The listing builds one solid part. Answer for the finished solid, in the listing's coordinates (mm). Face numbers are marked on the shaded views. A direction names the side the tool comes from. Coordinates: 2 decimals unless noted, no trailing zeros. Write each loop counter-clockwise with the first axis right and the second up, starting at its lowest first coordinate (ties: lowest second). Pieces come first, ordered by that corner, then holes.
from build123d import *

# Parameters (mm, degrees)
SKETCH1_W           = 200
SKETCH1_H           = 200
BOSS_EXTRUDE1_DEPTH = 5.6
SKETCH2_W           = 200
SKETCH2_H           = 200
SKETCH2_W_2         = 188.8
SKETCH2_H_2         = 188.8
BOSS_EXTRUDE2_DEPTH = 136
SKETCH3_W           = 5.6
SKETCH3_H           = 30.4
BOSS_EXTRUDE3_DEPTH = 32
FILLET1_R           = 25
SKETCH4_R           = 110
CUT_EXTRUDE1_DEPTH  = 12
FILLET3_R           = 10
FILLET2_R           = 2.4
SKETCH5_W           = 12
SKETCH5_H           = 12
BOSS_EXTRUDE4_DEPTH = 88
FILLET4_R           = 5
SKETCH6_R           = 1.55
CUT_EXTRUDE2_DEPTH  = 332.868889774
FILLET5_R           = 1.6


with BuildPart() as part:
    # Sketch1 → Boss-Extrude1 (new body)
    with BuildSketch(Plane(origin=(0, 0, 0), x_dir=(1, 0, 0), z_dir=(0, 1, 0))):
        with Locations((100, -100)):
            Rectangle(SKETCH1_W, SKETCH1_H)
    extrude(amount=BOSS_EXTRUDE1_DEPTH)

    # Sketch2 → Boss-Extrude2 (add)
    with BuildSketch(Plane(origin=(0, 5.6, 0), x_dir=(1, 0, 0), z_dir=(0, 1, 0))):
        with Locations((100, -100)):
            Rectangle(SKETCH2_W, SKETCH2_H)
        with Locations((100, -100)):
            Rectangle(SKETCH2_W_2, SKETCH2_H_2, mode=Mode.SUBTRACT)
    extrude(amount=BOSS_EXTRUDE2_DEPTH)

    # Sketch3 → Boss-Extrude3 (add)
    with BuildSketch(Plane(origin=(0, 141.6, 0), x_dir=(1, 0, 0), z_dir=(0, 1, 0))):
        with Locations((197.2, -100)):
            Rectangle(SKETCH3_W, SKETCH3_H)
    extrude(amount=BOSS_EXTRUDE3_DEPTH)

    # Fillet1
    fillet1_edges = [part.edges().sort_by_distance(p)[0] for p in [
        (197.2, 141.6, 115.2),
        (197.2, 141.6, 84.8),
    ]]
    fillet(fillet1_edges, radius=FILLET1_R)

    # Sketch4 → Cut-Extrude1 (cut)
    with BuildSketch(Plane.ZY):
        with Locations((100, 231.210075879)):
            Circle(SKETCH4_R)
    extrude(amount=-CUT_EXTRUDE1_DEPTH, mode=Mode.SUBTRACT)

    # Fillet3
    fillet3_edges = [part.edges().sort_by_distance(p)[0] for p in [
        (2.8, 141.6, 163.796820462),
        (2.8, 141.6, 36.203179538),
    ]]
    fillet(fillet3_edges, radius=FILLET3_R)

    # Fillet2
    fillet2_edges = [part.edges().sort_by_distance(p)[0] for p in [
        (0, 141.6, 16.541694665),
        (100, 141.6, 200),
        (200, 141.6, 170.1),
        (100, 141.6, 0),
        (100, 141.6, 194.4),
        (194.4, 141.6, 167.3),
        (100, 141.6, 5.6),
        (5.6, 141.6, 19.341694665),
        (194.4, 170.1, 84.8),
        (194.4, 170.1, 115.2),
        (200, 170.1, 115.2),
        (200, 170.1, 84.8),
        (200, 141.6, 29.9),
        (194.4, 141.6, 32.7),
        (200, 148.92233047, 122.52233047),
        (194.4, 148.92233047, 122.52233047),
        (194.4, 148.92233047, 77.47766953),
        (200, 148.92233047, 77.47766953),
        (5.6, 141.6, 180.658305335),
        (0, 141.6, 183.458305335),
        (0, 121.210075879, 100),
        (0, 141.16578268, 35.99814519),
        (0, 141.16578268, 164.00185481),
        (5.6, 121.210075879, 100),
        (5.6, 141.16578268, 35.99814519),
        (5.6, 141.16578268, 164.00185481),
    ]]
    fillet(fillet2_edges, radius=FILLET2_R)

    # Sketch5 → Boss-Extrude4 (add)
    with BuildSketch(Plane(origin=(0, 5.6, 0), x_dir=(1, 0, 0), z_dir=(0, 1, 0))):
        with Locations((188.4, -11.6)):
            Rectangle(SKETCH5_W, SKETCH5_H)
        with Locations((188.4, -188.4)):
            Rectangle(SKETCH5_W, SKETCH5_H)
        with Locations((11.6, -11.6)):
            Rectangle(SKETCH5_W, SKETCH5_H)
        with Locations((11.6, -188.4)):
            Rectangle(SKETCH5_W, SKETCH5_H)
    extrude(amount=BOSS_EXTRUDE4_DEPTH)

    # Fillet4
    fillet4_edges = [part.edges().sort_by_distance(p)[0] for p in [
        (182.4, 49.6, 17.6),
        (182.4, 49.6, 182.4),
        (17.6, 49.6, 17.6),
        (17.6, 49.6, 182.4),
    ]]
    fillet(fillet4_edges, radius=FILLET4_R)

    # Sketch6 → Cut-Extrude2 (cut, through all)
    with BuildSketch(Plane(origin=(200, 0, 0), x_dir=(0, 0, -1), z_dir=(1, 0, 0))):
        with Locations((-107.2, 167.2)):
            Circle(SKETCH6_R)
        with Locations((-92.8, 167.2)):
            Circle(SKETCH6_R)
    extrude(amount=-CUT_EXTRUDE2_DEPTH, mode=Mode.SUBTRACT)

    # Fillet5
    fillet5_edges = [part.edges().sort_by_distance(p)[0] for p in [
        (197.2, 173.6, 115.2),
        (194.4, 173.6, 100),
        (200, 173.6, 100),
        (197.2, 173.6, 84.8),
        (195.102943725, 173.6, 85.502943725),
        (199.297056275, 173.6, 85.502943725),
        (199.297056275, 173.6, 114.497056275),
        (195.102943725, 173.6, 114.497056275),
    ]]
    fillet(fillet5_edges, radius=FILLET5_R)


solid = part.part
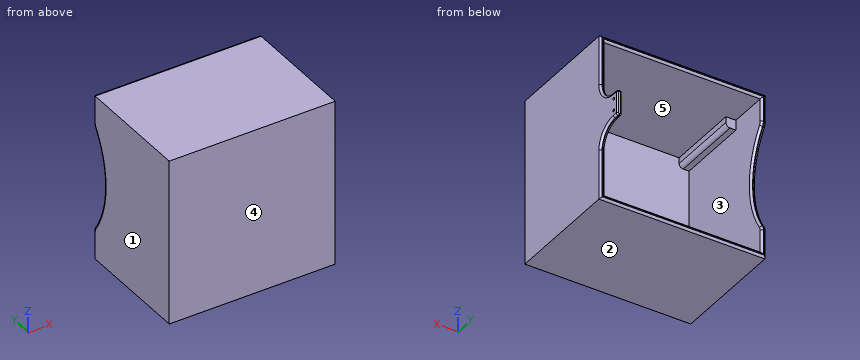
1. Section D-D on y = 111 is taken. Give the vertices of the cut face in (x, z).
Results found:
outline: (0, 0) - (200, 0) - (200, 200) - (0, 200) - close; hole (5.6, 5.6) - (194.4, 5.6) - (194.4, 194.4) - (5.6, 194.4) - close
2. Section B-B on x = 166.5 is taken. Give the vertices of the cut face in (y, z).
Results found:
outline: (0, 0) - (139.2, 0) arc R2.4 ccw to (141.6, 2.4) - (141.6, 3.2) arc R2.4 ccw to (139.2, 5.6) - (5.6, 5.6) - (5.6, 194.4) - (139.2, 194.4) arc R2.4 ccw to (141.6, 196.8) - (141.6, 197.6) arc R2.4 ccw to (139.2, 200) - (0, 200) - close
3. Flat-ended cylindrical pins translate along their axes: P1, Ø8, axis at x = 161, z = 84.5, coming from the +Y side; P2, Ø9.5, axis at x = 189, z = 10.5, coming from the +Y side; P3, Ø0.6, axis at x = 197.5, y = 168.5, coming from the -Z side; P4, Ø5, axis at x = 171, z = 134.5, coming from the -Y side. Find the tip coordinate at first contact, or state that the pin passes through.
Results found:
P1: stops at y = 5.6
P2: stops at y = 93.6
P3: stops at z = 84.8
P4: stops at y = 0
4. A tool of negligible diameter and unlimited length cuts with its end or side. For the marked faces 4 and 5, from which of +Z, -Z, +X, -X, +Y, -Y can it reach the whole face along a straight path? Write none if from no direction.
Results found:
face 4: +Z, -Z, +X, -X, -Y
face 5: +Y
5. Section C-C on z = 179 is taken. Give the vertices of the cut face in (x, y).
Results found:
outline: (0, 0) - (200, 0) - (200, 139.2) arc R2.4 ccw to (197.6, 141.6) - (196.8, 141.6) arc R2.4 ccw to (194.4, 139.2) - (194.4, 5.6) - (5.6, 5.6) - (5.6, 139.2) arc R2.4 ccw to (3.2, 141.6) - (2.4, 141.6) arc R2.4 ccw to (0, 139.2) - close
6. Find the intervals of material crossed by L1, parallel to Z at x = 197, y = 167; L2, parallel to X at y = 79.5, z = 66.5; L3, parallel to Y at x = 196.05, z = 107.2, in increasing order.
Results found:
L1: z = 84.8 to 91.26, 94.34 to 105.66, 108.74 to 115.2
L2: x = 0 to 5.6, 194.4 to 200
L3: y = 0 to 165.65, 168.75 to 173.6
7. For a pull along X with two mould halves and no side action, classify the marked faces 1, 2 and 3 as pulls with the +X half, pulls with the -X half, needs draft (parallel to the pull), parting line crosses it, or undercut.
Results found:
face 1: pulls with the -X half
face 2: needs draft
face 3: undercut
8. Section A-A on y = 66.5 is taken. Give the vertices of the cut face in (x, z), then the cut area to 3 significant figures.
Results found:
outline: (0, 0) - (200, 0) - (200, 200) - (0, 200) - close; hole (5.6, 17.6) - (12.6, 17.6) arc R5 cw to (17.6, 12.6) - (17.6, 5.6) - (182.4, 5.6) - (182.4, 12.6) arc R5 cw to (187.4, 17.6) - (194.4, 17.6) - (194.4, 182.4) - (187.4, 182.4) arc R5 cw to (182.4, 187.4) - (182.4, 194.4) - (17.6, 194.4) - (17.6, 187.4) arc R5 cw to (12.6, 182.4) - (5.6, 182.4) - close
area: 4,910 mm2
